CAD build for the part. Positions are in the model's coordinates, mm. Coordinates: 2 decimals unless noted, no trailing zeros. Write each loop counter-clockwise with the first axis right and the second up, starting at its lowest first coordinate (ties: lowest second). Pieces come first, ordered by that corner, then holes. Notation, with made-up numbers: (21.5, -17) - (58.5, -17) arc R28 ccw to (58.5, 18) - close; hole circle Ø10 at (81, -32). An arc over 180 degrees is marked (long way). Answer in a Markdown table with one row per item. Add a question column.
Q1. Band-saw the part on B-B (z = 1.25). List the corners of the cut face in (x, y).
Q2. Band-saw the part on D-D (y = -39.5). List the corners of the cut face in (x, z), and give its area (3 significant figures).
Q3. Band-saw the part on A-A (y = -126.27). List the corners of the cut face in (x, z).
Q4. Drill centre lines: line 1 along X through (y, z) = (-126.27, 5.9); line 2 along X through (y, z) = (-104, 6.25); line 3 along X through (y, z) = (-130.5, 3). Where is each one in solid material? Low to high. Write a range as from..to.
Q5. Pin check, flat tips, straight feed: pin 1 (1.5 mm diameter, centred on x = 5.5, y = -54, fed in from -Z); pin 2 (4.5 mm diameter, centred on x = -2.5, z = 1, fed in from -Y). Stop position of each tip, or through.
Q6. Band-saw the part on C-C (y = 10.95). List the corners of the cut face in (x, z), and give its area (3 significant figures).
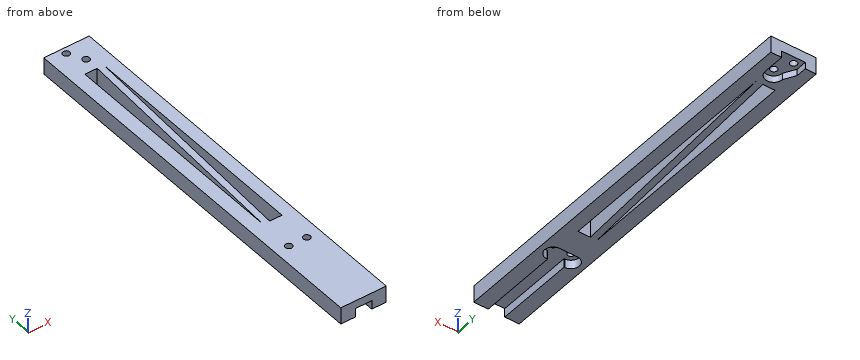
```python
from build123d import *

# Parameters (mm, degrees)
PAD_DEPTH            = 3
PAD001_DEPTH         = 4.65
SKETCH002_R          = 1.58
POCKET_DEPTH         = 0.001
POCKET_DEPTH_BACK    = -7.651
POCKET001_DEPTH      = 0.001
POCKET001_DEPTH_BACK = -7.651
POCKET002_DEPTH      = 4
SKETCH005_R          = 1.58
POCKET003_DEPTH      = 0.001
POCKET003_DEPTH_BACK = -7.651


with BuildPart() as part:
    # Sketch → Pad (new body)
    with BuildSketch(Plane.XY):
        with BuildLine():
            ThreePointArc((-3.95, 3.95), (0, 0), (3.95, 3.95))
            Line((3.95, 13.95), (3.95, 3.95))
            Line((3.95, 13.95), (8.95, 13.95))
            Line((8.95, 13.95), (8.95, 0))
            Line((8.95, 0), (8.95, -166.05))
            Line((8.95, -166.05), (-11.8411, -166.05))
            Line((-11.8411, -166.05), (-11.8411, 0))
            Line((-11.8411, 13.95), (-11.8411, 0))
            Line((-6.8411, 13.95), (-11.8411, 13.95))
            Line((-6.8411, 13.95), (-6.8411, 9.04))
            Line((-6.8411, 9.04), (-3.95, 3.95))
        make_face()
    extrude(amount=PAD_DEPTH)

    # Sketch001 → Pad001 (join)
    with BuildSketch(Plane.XY.offset(3)):
        Polygon((-11.8411, 0), (-11.8411, 13.95), (0, 13.95), (8.95, 13.95), (8.95, 0), (8.95, -166.05), (-11.8411, -166.05), align=None)
    extrude(amount=PAD001_DEPTH)

    # Sketch002 → Pocket (cut, two sides)
    with BuildSketch(Plane(origin=(0, 0.2, 0), x_dir=(1, 0, 0), z_dir=(0, 0, 1))) as pocket_sk:
        with Locations((0, 3.75)):
            Circle(SKETCH002_R)
        with Locations((-3.75, 10.75)):
            Circle(SKETCH002_R)
    extrude(amount=-POCKET_DEPTH, mode=Mode.SUBTRACT)
    extrude(pocket_sk.sketch, amount=-POCKET_DEPTH_BACK, mode=Mode.SUBTRACT)

    # Sketch003 → Pocket001 (cut, two sides)
    with BuildSketch(Plane.XY) as pocket001_sk:
        Polygon((0.11, -2.63), (-5.54, -2.63), (-5.54, -110.63), align=None)
        Polygon((-2.54, -110.63), (3.11, -110.63), (3.11, -2.63), align=None)
    extrude(amount=-POCKET001_DEPTH, mode=Mode.SUBTRACT)
    extrude(pocket001_sk.sketch, amount=-POCKET001_DEPTH_BACK, mode=Mode.SUBTRACT)

    # Sketch004 → Pocket002 (cut)
    with BuildSketch(Plane.XY):
        with BuildLine():
            Line((-5.22555, -130.05), (-5.22555, -166.05))
            Line((-5.22555, -166.05), (2.33445, -166.05))
            Line((2.33445, -166.05), (2.33445, -130.05))
            Line((2.33445, -130.05), (2.67, -130.05))
            ThreePointArc((2.67, -130.05), (6.45, -126.27), (2.67, -122.49))
            Line((-5.5611, -122.49), (2.67, -122.49))
            ThreePointArc((-5.5611, -122.49), (-9.3411, -126.27), (-5.5611, -130.05))
            Line((-5.22555, -130.05), (-5.5611, -130.05))
        make_face()
    extrude(amount=POCKET002_DEPTH, mode=Mode.SUBTRACT)

    # Sketch005 → Pocket003 (cut, two sides)
    with BuildSketch(Plane.XY) as pocket003_sk:
        with Locations((-5.5611, -126.27)):
            Circle(SKETCH005_R)
        with Locations((2.67, -126.27)):
            Circle(SKETCH005_R)
    extrude(amount=-POCKET003_DEPTH, mode=Mode.SUBTRACT)
    extrude(pocket003_sk.sketch, amount=-POCKET003_DEPTH_BACK, mode=Mode.SUBTRACT)


solid = part.part
```
Checked values:
| question | item | result |
|---|---|---|
| 1 | outline | (-11.84, -166.05) - (-5.23, -166.05) - (-5.23, -130.05) - (-5.56, -130.05) arc R3.78 cw to (-5.56, -122.49) - (2.67, -122.49) arc R3.78 cw to (2.67, -130.05) - (2.33, -130.05) - (2.33, -166.05) - (8.95, -166.05) - (8.95, 13.95) - (3.95, 13.95) - (3.95, 3.95) arc R3.95 cw to (-3.95, 3.95) - (-6.84, 9.04) - (-6.84, 13.95) - (-11.84, 13.95) - close; hole (-5.54, -110.63) - (0.11, -2.63) - (-5.54, -2.63) - close; hole (-2.54, -110.63) - (3.11, -110.63) - (3.11, -2.63) - close |
| 2 | outline | (-11.84, 0) - (-5.54, 0) - (-5.54, 7.65) - (-11.84, 7.65) - close; (-1.82, 0) - (1.18, 0) - (1.18, 7.65) - (-1.82, 7.65) - close; (3.11, 0) - (8.95, 0) - (8.95, 7.65) - (3.11, 7.65) - close |
| 2 | area | 116 mm² |
| 3 | outline | (-11.84, 0) - (-9.34, 0) - (-9.34, 4) - (-7.14, 4) - (-7.14, 7.65) - (-11.84, 7.65) - close; (-3.98, 4) - (1.09, 4) - (1.09, 7.65) - (-3.98, 7.65) - close; (4.25, 4) - (6.45, 4) - (6.45, 0) - (8.95, 0) - (8.95, 7.65) - (4.25, 7.65) - close |
| 4 | line 1 | x = -11.84..-7.14, -3.98..1.09, 4.25..8.95 |
| 4 | line 2 | x = -11.84..-5.54, -5.19..-2.19, 3.11..8.95 |
| 4 | line 3 | x = -11.84..-5.23, 2.33..8.95 |
| 5 | pin 1 | stops at z = 0 |
| 5 | pin 2 | stops at y = -122.49 |
| 6 | outline | (-11.84, 0) - (-6.84, 0) - (-6.84, 3) - (-5.33, 3) - (-5.33, 7.65) - (-11.84, 7.65) - close; (-2.17, 3) - (3.95, 3) - (3.95, 0) - (8.95, 0) - (8.95, 7.65) - (-2.17, 7.65) - close |
| 6 | area | 112 mm² |
